from build123d import *

# Parameters (mm, degrees)
SKETCH1_R           = 51.3588
BOSS_EXTRUDE1_DEPTH = 165.1
DOME1_FACE_RADIUS   = 51.3588
DOME1_HEIGHT        = 50.8


# Read off the part's stored shape, not the designer's step: Shell1
with BuildPart() as part:
    # Sketch1 → Boss-Extrude1 (new body)
    with BuildSketch(Plane(origin=(0, 0, 0), x_dir=(1, 0, 0), z_dir=(0, 1, 0))):
        with Locations(Location((0, 0, 0), (0, 0, 270))):
            Circle(SKETCH1_R)
    extrude(amount=BOSS_EXTRUDE1_DEPTH)

    # Dome1: a dome of height H over a round flat face of radius A is a cap of a sphere of radius (A * A + H * H) / (2 * H)
    dome1_r = (DOME1_FACE_RADIUS * DOME1_FACE_RADIUS + DOME1_HEIGHT * DOME1_HEIGHT) / (2 * DOME1_HEIGHT)
    dome1_base = Plane((0, 165.1, 0), z_dir=(0, 1, 0))
    with Locations(dome1_base.offset(DOME1_HEIGHT - dome1_r)):
        dome1_ball = Sphere(dome1_r, mode=Mode.PRIVATE)
    add(split(dome1_ball, bisect_by=dome1_base, keep=Keep.TOP, mode=Mode.PRIVATE))

    # Shell1 outline → Shell1 (revolve, cut)
    with BuildSketch(Plane.XY):
        with BuildLine():
            Line((50.8, 0), (50.800000001, 165.096935001))
            ThreePointArc((50.800000001, 165.096935001), (35.725082804, 200.65835259), (0, 215.3412))
            Line((0, 215.3412), (0, 0))
            Line((0, 0), (50.8, 0))
        make_face()
    revolve(axis=Axis((0, 0, 0), (0, 1, 0)), mode=Mode.SUBTRACT)


solid = part.part
CAD build for the part. Positions are in the model's coordinates, mm. Coordinates: 2 decimals unless noted, no trailing zeros. Order: outer loops, then holes, each group sorted by start corner. A loop starts at its lowest first (then second) coordinate and runs counter-clockwise, first axis right, second up.
Item 1: Band-saw the part on B-B on y = 76. List the corners of the cut face in (x, z).
Check sheet entries:
outline: circle Ø102.72 at (0, 0); hole circle Ø101.6 at (0, 0)
Item 2: Band-saw the part on C-C on x = 0. List the corners of the cut face in (y, z).
Check sheet entries:
outline: (0, -51.36) - (165.1, -51.36) arc R51.36 ccw to (165.1, 51.36) - (0, 51.36) - (0, 50.8) - (165.1, 50.8) arc R50.8 cw to (165.1, -50.8) - (0, -50.8) - close
Item 3: Pin check, flat tips, straight feed: pin 1 Ø4 at (y, z) = (189, 8) entering from -X; pin 2 Ø6 at (x, y) = (26, 151.5) entering from +Z; pin 3 Ø5 at (y, z) = (160.5, -25.5) entering from +X. Stop position of each tip, or through.
Check sheet entries:
pin 1: stops at x = -45.55
pin 2: stops at z = 45.92
pin 3: stops at x = 45.92
Item 4: Band-saw the part on A-A on z = 0. List the corners of the cut face in (x, y).
Check sheet entries:
outline: (-51.36, 0) - (-50.8, 0) - (-50.8, 165.1) arc R50.8 cw to (50.8, 165.1) - (50.8, 0) - (51.36, 0) - (51.36, 165.1) arc R51.36 ccw to (-51.36, 165.1) - close
Item 5: Drill centre lines: L1, parallel to X at y = 80.5, z = 0; L2, parallel to Z at x = -28, y = 125; L3, parallel to Z at x = -10.5, y = 124.5. Where is each one in solid material? Low to high.
Check sheet entries:
L1: x = -51.36 to -50.8, 50.8 to 51.36
L2: z = -43.05 to -42.39, 42.39 to 43.05
L3: z = -50.27 to -49.7, 49.7 to 50.27
Item 6: Two-plate mould, pull along X, no slides. Class faces 1 (the face through (-45.564, 81.394, 23.699)), 2 (the face through (49.7, 0, -11.7)), 3 (the face through (-11.012, 83.704, 49.592)): +X half, -X half, draft (parallel to the pull), parting line (faces both ways), or undercut.
Check sheet entries:
face 1: parting line
face 2: draft
face 3: undercut
